Autodesk Inventor part; units mm, degrees
ref_plane "YZ Plane" through (0, 0, 0) normal (1, 0, 0) x (0, 1, 0)
ref_plane "XZ Plane" through (0, 0, 0) normal (0, 1, 0) x (-1, 0, 0)
ref_plane "XY Plane" through (0, 0, 0) normal (0, 0, 1) x (1, 0, 0)
sketch "スケッチ1" plane through (0, 0, 0) normal (0, 0, 1) x (1, 0, 0)
  line L0 (-68, 0) -> (68, 0) construction
  line L1 (-68, -16.2338) -> (68, -16.2338)
  line L2 (68, 16.2338) -> (-68, 16.2338)
  arc A0 (-68, 16.2338) -> (-68, -16.2338) centre (-68, 0) ccw
  arc A1 (68, -16.2338) -> (68, 16.2338) centre (68, 0) ccw
  line L3 (-68, -16.6528) -> (68, -16.6528)
  arc A2 (68, -16.6528) -> (68, 16.6528) centre (68, 0) ccw
  line L4 (68, 16.6528) -> (-68, 16.6528)
  arc A3 (-68, 16.6528) -> (-68, -16.6528) centre (-68, 0) ccw
  line L5 (-68, -15.8528) -> (68, -15.8528)
  arc A4 (68, -15.8528) -> (68, 15.8528) centre (68, 0) ccw
  line L6 (68, 15.8528) -> (-68, 15.8528)
  arc A5 (-68, 15.8528) -> (-68, -15.8528) centre (-68, 0) ccw
  point P0 (0, 0)
  dimension "d0" = 136
  dimension "d1" = 16.2338
  dimension "d2" = 0.419
  dimension "d3" = 0.8
extrude "押し出し1" add sketch "スケッチ1" along normal mid plane 6 contours A0 L2 A1 L1 | A3 L4 A2 L3
properties part number "belt4" material "ゴム"
For this review, take the finished solid that the model builds, in its own axes (mm). A direction names the side the tool comes from. Round coordinates to 2 decimals unless told otherwise and drop trailing zeros. Write each loop counter-clockwise with the first axis right and the second up, starting at its lowest first coordinate (ties: lowest second). Pieces come first, ordered by that corner, then holes. Notation, with made-up numbers: (78, -20) -> (118, -20) arc R13 ccw to (118, -6) -> close; hole circle Ø5 at (0.25, 37). An arc over 180 degrees is marked (long way). One line per question, with ' | ' between items. Start each with the question number.
(1) Mouldability with a two-part tool opening along X and no side actions: class faces 1 (the face through (83.85, -0.35, 0.04)), 2 (the face through (84.65, -0.37, 0.04)), 3 (the face through (-0.4, 16.1, -3)), 4 (the face through (-84.65, 0.37, 0.04)) as released by +X, released by -X, zero draft, split by the parting line, or undercut.
(2) For line 1 along Y through (x, z) = (6.5, -1.5); line 2 along X through (y, z) = (9, 2.4); line 3 along Y through (x, z) = (77, -1.9), list the stretches that pass through material, from the lowest coordinate up. Write a range as from..to.
(3) Add section A-A, the plane y = 0. Write out the cut boundary in (x, z), plus the area to 3 significant figures.
(4) Tool access review of faces 5 (the face through (-1, -16.653, 0)), 6 (the face through (-83.85, 0.35, 0.04)): name each direction out of +Z, -Z, +X, -X, +Y, -Y from which nothing blocks a thin tool from reaching the whole face with its end or side.
(5) Add section B-B, the plane x = -62. Write out the cut boundary in (y, z), plus the area to 3 significant figures.
(6) Add section C-C, the plane z = 1.1. Write out the cut boundary in (x, y).
Answer list:
1) face 1: undercut | face 2: released by +X | face 3: zero draft | face 4: released by -X
2) line 1: -16.65..-15.85, 15.85..16.65 | line 2: -82.01..-81.05, 81.05..82.01 | line 3: -14.01..-13.05, 13.05..14.01
3) outline: (-84.65, -3) -> (-83.85, -3) -> (-83.85, 3) -> (-84.65, 3) -> close; (83.85, -3) -> (84.65, -3) -> (84.65, 3) -> (83.85, 3) -> close | area: 9.60 mm²
4) face 5: +Z, -Z, +X, -X, -Y | face 6: +Z, -Z
5) outline: (-16.65, -3) -> (-15.85, -3) -> (-15.85, 3) -> (-16.65, 3) -> close; (15.85, -3) -> (16.65, -3) -> (16.65, 3) -> (15.85, 3) -> close | area: 9.60 mm²
6) outline: (-68, -16.65) -> (68, -16.65) arc R16.65 ccw to (68, 16.65) -> (-68, 16.65) arc R16.65 ccw to start; hole (-68, -15.85) -> (68, -15.85) arc R15.85 ccw to (68, 15.85) -> (-68, 15.85) arc R15.85 ccw to start
